```python
from build123d import *

# Parameters (mm, degrees)
MODEL_R             = 1.775
MODEL_W             = 6.859999999
MODEL_H             = 15
MODEL_W_2           = 6.860000001
BOSS_EXTRUDE1_DEPTH = 6.6


with BuildPart() as part:
    # Model → Boss-Extrude1 (new body)
    with BuildSketch(Plane.XY):
        with BuildLine():
            Line((213.279999903, 109.659999999), (2.000000001, 109.659999999))
            ThreePointArc((2.000000001, 109.659999999), (0.585786439, 109.074213562), (0, 107.660000001))
            Line((0, 107.660000001), (0, 2.000000001))
            ThreePointArc((0, 2.000000001), (0.585786438, 0.585786438), (2.000000001, 0))
            Line((2.000000001, 0), (213.279999903, 0))
            ThreePointArc((213.279999903, 0), (214.694213466, 0.585786438), (215.279999904, 2.000000001))
            Line((215.279999904, 2.000000001), (215.279999904, 107.660000001))
            ThreePointArc((215.279999904, 107.660000001), (214.694213465, 109.074213562), (213.279999903, 109.659999999))
        make_face()
        with Locations((10.31, 83.101155497)):
            Circle(MODEL_R, mode=Mode.SUBTRACT)
        with Locations((10.31, 26.551155498)):
            Circle(MODEL_R, mode=Mode.SUBTRACT)
        with Locations((204.970000001, 26.551155498)):
            Circle(MODEL_R, mode=Mode.SUBTRACT)
        with Locations((204.970000001, 83.101155497)):
            Circle(MODEL_R, mode=Mode.SUBTRACT)
        with Locations((204.97, 54.826155497)):
            Rectangle(MODEL_W, MODEL_H, mode=Mode.SUBTRACT)
        with Locations((10.31, 54.826155497)):
            Rectangle(MODEL_W_2, MODEL_H, mode=Mode.SUBTRACT)
    extrude(amount=BOSS_EXTRUDE1_DEPTH)


solid = part.part
```
Verification items for the finished model (mm, model axes). A direction names the side the tool comes from. Round coordinates to 2 decimals unless told otherwise and drop trailing zeros. Order: outer loops, then holes, each group sorted by start corner. A loop starts at its lowest first (then second) coordinate and runs counter-clockwise, first axis right, second up.
1) Cross-section at A-A, the plane y = 51. Record the cut outline in (x, z), plus the area to 3 significant figures.
Geometry says:
outline: (0, 0) - (6.88, 0) - (6.88, 6.6) - (0, 6.6) - close; (13.74, 0) - (201.54, 0) - (201.54, 6.6) - (13.74, 6.6) - close; (208.4, 0) - (215.28, 0) - (215.28, 6.6) - (208.4, 6.6) - close
area: 1,330 mm2
2) Material ranges on line 1 (Y direction, x = 10.31, z = 3.5); line 2 (X direction, y = 59, z = 2.75); line 3 (X direction, y = 82, z = 6.25), recorded low to high.
Geometry says:
line 1: y = 0 to 24.78, 28.33 to 47.33, 62.33 to 81.33, 84.88 to 109.66
line 2: x = 0 to 6.88, 13.74 to 201.54, 208.4 to 215.28
line 3: x = 0 to 8.92, 11.7 to 203.58, 206.36 to 215.28
3) Tool access check on faces 5 (the flat face through (106, 56, 0)), 6 (the flat face through (208.4, 55, 3)). Record the directions out of +Z, -Z, +X, -X, +Y, -Y that give a thin tool (end or side, any length) a straight path to the whole face; none if there is none.
Geometry says:
face 5: -Z, +X, -X, +Y, -Y
face 6: +Z, -Z
4) Depth check by flat-ended pin: pin 1 (5.5 mm diameter, centred on x = 10.31, y = 26.55, fed in from -Z). Enter the tip coordinate at first touch or a pass-through.
Geometry says:
pin 1: stops at z = 0
5) Draft check along X on faces 1 (the flat face through (215.28, 54, 3)), 2 (the flat face through (205, 62.326, 3)), 3 (the flat face through (0, 56, 3)), 4 (the flat face through (106, 56, 6.6)). Enter one of: +X half, -X half, draft (parallel to the pull), parting line (faces both ways), or undercut.
Geometry says:
face 1: +X half
face 2: undercut
face 3: -X half
face 4: draft
